Read the model definition and answer for the solid it produces. Units are mm, in the model's axes. Round coordinates to 2 decimals unless told otherwise and drop trailing zeros. Write each loop counter-clockwise with the first axis right and the second up, starting at its lowest first coordinate (ties: lowest second). Pieces come first, ordered by that corner, then holes. Notation, with made-up numbers: (12.5, 7) - (42.5, 7) arc R28 cw to (42.5, 37) - close; hole circle Ø6 at (-16, -7.5). An arc over 180 degrees is marked (long way). Use one line per item in the form item = value. Start each with the question number.
1) This flat-tipped pin is pushed along its axis until it touches: pin 1 (2.5 mm diameter, centred on x = -171, z = -27, fed in from +Y). Where does it stop, or does it pass through?
2) The part is cut by section B-B, the plane x = -131.5. Give the vertices of the cut face in (y, z).
3) Consider line 1 along X through (y, z) = (1.05, -173); line 2 along Z through (x, y) = (-111, 0.8); line 3 along Z through (x, y) = (-29, 1.45). Determine where each line is inside the solid, lowest interval first. Write a range as from..to.
4) For a pull along X with two mould halves and no side action, classify faces 1 (the face through (-139.239, 1.521, -107.096)), 2 (the face through (-99, 0, -99)) as released by +X, released by -X, zero draft, split by the parting line, or undercut.
5) The part is cut by section A-A, the plane y = 0.6. Count the separate pieces of the cut face and the enclosed holes in it, plus the area to 3 significant figures.
Autodesk Inventor part; units mm, degrees
ref_plane "YZ Plane" through (0, 0, 0) normal (1, 0, 0) x (0, 1, 0)
ref_plane "XZ Plane" through (0, 0, 0) normal (0, 1, 0) x (-1, 0, 0)
ref_plane "XY Plane" through (0, 0, 0) normal (0, 0, 1) x (1, 0, 0)
sketch "Sketch1" plane through (0, 0, 0) normal (0, 1, 0) x (-1, 0, 0)
  line L0 (0, 0) -> (200, 0)
  line L1 (200, 0) -> (200, -200)
  line L2 (200, -200) -> (0, -200)
  line L3 (0, -200) -> (0, 0)
  dimension "d0" = 200
  dimension "d1" = 200
extrude "Extrusion1" add sketch "Sketch1" along normal blind 3
sketch "Sketch4" plane through (0, 3, 0) normal (0, 1, 0) x (1, 0, 0)
  line L0 (-175, 37) -> (-175, 40)
  line L1 (-175, 40) -> (-85, 40)
  line L2 (-85, 40) -> (-85, 37)
  line L3 (-85, 37) -> (-175, 37)
  line L4 (-190, 6) -> (-10, 6)
  line L5 (-200, 200) -> (-200, 0)
  line L6 (-175, 160) -> (-175, 163)
  line L7 (-175, 163) -> (-85, 163)
  line L8 (-85, 163) -> (-85, 160)
  line L9 (-85, 160) -> (-175, 160)
  line L10 (0, 0) -> (0, 200)
  line L11 (-10, 194) -> (-190, 194)
  dimension "d24" = 3
  dimension "d25" = 90
  dimension "d26" = 31
  dimension "d27" = 25
  dimension "d28" = 3
  dimension "d29" = 120
  dimension "d30" = 25
  dimension "d31" = 85
  dimension "d52" = 31
extrude "Extrusion4" cut sketch "Sketch4" against normal blind 3
sketch "Sketch5" plane through (0, 3, 0) normal (0, 1, 0) x (1, 0, 0)
  circle A0 centre (-131.5, 100) radius 10.5
  line L0 (-200, 200) -> (-200, 0)
  line L1 (-175, 40) -> (-85, 40)
  line L2 (-175, 160) -> (-175, 163)
  line L3 (-85, 160) -> (-175, 160)
  point P0 (0, 0)
  dimension "d34" = 21
  dimension "d37" = 60
  dimension "d40" = 43.5
  dimension "d53" = 60
extrude "Extrusion5" cut sketch "Sketch5" against normal blind 10
sketch "Sketch8" plane through (0, 3, 0) normal (0, 1, 0) x (1, 0, 0)
  circle A0 centre (-131.5, 100) radius 10.5
  point P0 (0, 0)
sketch "Sketch11" plane through (0, 3, 0) normal (0, 1, 0) x (1, 0, 0)
  line L0 (-111, 108.75) -> (-111, 91.25)
  circle A0 centre (-131.5, 100) radius 10.5
  circle A1 centre (-111, 108.75) radius 1.5
  circle A2 centre (-111, 91.25) radius 1.5
  point P0 (0, 0)
  dimension "d60" = 20.5
  dimension "d61" = 3
  dimension "d62" = 3
  dimension "d63" = 17.5
  dimension "d64" = 8.75
extrude "Extrusion8" cut sketch "Sketch11" against normal blind 10 contours A2 | A1
sketch "Sketch12" plane through (0, 3, 0) normal (0, 1, 0) x (1, 0, 0)
  circle A0 centre (-171, 27) radius 1.6
  line L0 (-194, 190) -> (-194, 10)
  line L1 (-190, 6) -> (-10, 6)
  circle A1 centre (-171, 173) radius 1.6
  line L2 (-10, 194) -> (-190, 194)
  circle A2 centre (-29, 27) radius 1.6
  line L3 (-6, 10) -> (-6, 190)
  circle A3 centre (-29, 173) radius 1.6
  point P0 (0, 0)
  dimension "d67" = 3.2
  dimension "d68" = 23
  dimension "d69" = 21
  dimension "d70" = 3.2
  dimension "d71" = 21
  dimension "d72" = 23
  dimension "d73" = 3.2
  dimension "d74" = 21
  dimension "d75" = 23
  dimension "d76" = 3.2
  dimension "d77" = 21
  dimension "d78" = 23
extrude "Extrusion9" cut sketch "Sketch12" against normal blind 10
equation "\"d26\" = d52"
equation "\"d37\" = d53"
properties part number "Part 1 base"
Geometry results:
q1.pin_1 = through
q2.outline = (0, -200) - (3, -200) - (3, -163) - (0, -163) - close; (0, -160) - (3, -160) - (3, -110.5) - (0, -110.5) - close; (0, -89.5) - (3, -89.5) - (3, -40) - (0, -40) - close; (0, -37) - (3, -37) - (3, 0) - (0, 0) - close
q3.line_1 = -200..-172.6, -169.4..-30.6, -27.4..0
q3.line_2 = -200..-163, -160..-110.25, -107.25..-92.75, -89.75..-40, -37..0
q3.line_3 = -200..-174.6, -171.4..-28.6, -25.4..0
q4.face_1 = undercut
q4.face_2 = zero draft
q5.separate_pieces = 1
q5.enclosed_holes = 9
q5.area = 39,100 mm2
